Geometry check sheet. Reference: the model listing, model coordinates, mm. A direction names the side the tool comes from. Round coordinates to 2 decimals unless told otherwise and drop trailing zeros. Order: outer loops, then holes, each group sorted by start corner. A loop starts at its lowest first (then second) coordinate and runs counter-clockwise, first axis right, second up.
```python
from build123d import *

# Parameters (mm, degrees)
F1_DEPTH = 6


with BuildPart() as f1:
    # F0 (on Top) → F1 (new body)
    with BuildSketch(Plane.XY):
        with BuildLine():
            Line((38, 4), (-38, 4))
            ThreePointArc((-38, 4), (-42, 0), (-38, -4))
            Line((-38, -4), (38, -4))
            Line((38, -4), (42, 0))
            Line((42, 0), (38, 4))
        make_face()
        with BuildLine():
            ThreePointArc((-33.612533, 2.35), (-32.899958, 1.269741), (-32.65, 0))
            ThreePointArc((-32.65, 0), (-32.899958, -1.269741), (-33.612533, -2.35))
            ThreePointArc((-33.612533, -2.35), (-36, -3.35), (-38.387467, -2.35))
            ThreePointArc((-38.387467, -2.35), (-39.35, 0), (-38.387467, 2.35))
            ThreePointArc((-38.387467, 2.35), (-36, 3.35), (-33.612533, 2.35))
        make_face(mode=Mode.SUBTRACT)
        with BuildLine():
            ThreePointArc((-25.654792, 2.25), (-24.98467, 1.212554), (-24.75, 0))
            ThreePointArc((-24.75, 0), (-24.98467, -1.212554), (-25.654792, -2.25))
            ThreePointArc((-25.654792, -2.25), (-28, -3.25), (-30.345208, -2.25))
            ThreePointArc((-30.345208, -2.25), (-31.25, 0), (-30.345208, 2.25))
            ThreePointArc((-30.345208, 2.25), (-28, 3.25), (-25.654792, 2.25))
        make_face(mode=Mode.SUBTRACT)
        with BuildLine():
            ThreePointArc((-17.697827, 2.15), (-17.069612, 1.155564), (-16.85, 0))
            ThreePointArc((-16.85, 0), (-17.069612, -1.155564), (-17.697827, -2.15))
            ThreePointArc((-17.697827, -2.15), (-20, -3.15), (-22.302173, -2.15))
            ThreePointArc((-22.302173, -2.15), (-23.15, 0), (-22.302173, 2.15))
            ThreePointArc((-22.302173, 2.15), (-20, 3.15), (-17.697827, 2.15))
        make_face(mode=Mode.SUBTRACT)
        with BuildLine():
            ThreePointArc((-9.741682, 2.05), (-9.154796, 1.098779), (-8.95, 0))
            ThreePointArc((-8.95, 0), (-9.154796, -1.098779), (-9.741682, -2.05))
            ThreePointArc((-9.741682, -2.05), (-12, -3.05), (-14.258318, -2.05))
            ThreePointArc((-14.258318, -2.05), (-15.05, 0), (-14.258318, 2.05))
            ThreePointArc((-14.258318, 2.05), (-12, 3.05), (-9.741682, 2.05))
        make_face(mode=Mode.SUBTRACT)
        with BuildLine():
            ThreePointArc((-1.786406, 1.95), (-1.240235, 1.042208), (-1.05, 0))
            ThreePointArc((-1.05, 0), (-1.240235, -1.042208), (-1.786406, -1.95))
            ThreePointArc((-1.786406, -1.95), (-4, -2.95), (-6.213594, -1.95))
            ThreePointArc((-6.213594, -1.95), (-6.95, 0), (-6.213594, 1.95))
            ThreePointArc((-6.213594, 1.95), (-4, 2.95), (-1.786406, 1.95))
        make_face(mode=Mode.SUBTRACT)
        with BuildLine():
            ThreePointArc((6.167948, 1.85), (6.674056, 0.985862), (6.85, 0))
            ThreePointArc((6.85, 0), (6.674056, -0.985862), (6.167948, -1.85))
            ThreePointArc((6.167948, -1.85), (4, -2.85), (1.832052, -1.85))
            ThreePointArc((1.832052, -1.85), (1.15, 0), (1.832052, 1.85))
            ThreePointArc((1.832052, 1.85), (4, 2.85), (6.167948, 1.85))
        make_face(mode=Mode.SUBTRACT)
        with BuildLine():
            ThreePointArc((14.12132, 1.75), (14.588062, 0.92975), (14.75, 0))
            ThreePointArc((14.75, 0), (14.588062, -0.92975), (14.12132, -1.75))
            ThreePointArc((14.12132, -1.75), (12, -2.75), (9.87868, -1.75))
            ThreePointArc((9.87868, -1.75), (9.25, 0), (9.87868, 1.75))
            ThreePointArc((9.87868, 1.75), (12, 2.75), (14.12132, 1.75))
        make_face(mode=Mode.SUBTRACT)
        with BuildLine():
            ThreePointArc((22.073644, 1.65), (22.501765, 0.873883), (22.65, 0))
            ThreePointArc((22.65, 0), (22.501765, -0.873883), (22.073644, -1.65))
            ThreePointArc((22.073644, -1.65), (20, -2.65), (17.926356, -1.65))
            ThreePointArc((17.926356, -1.65), (17.35, 0), (17.926356, 1.65))
            ThreePointArc((17.926356, 1.65), (20, 2.65), (22.073644, 1.65))
        make_face(mode=Mode.SUBTRACT)
        with BuildLine():
            ThreePointArc((30, 1.5), (30.371708, 0.790569), (30.5, 0))
            ThreePointArc((30.5, 0), (30.371708, -0.790569), (30, -1.5))
            ThreePointArc((30, -1.5), (28, -2.5), (26, -1.5))
            ThreePointArc((26, -1.5), (25.5, 0), (26, 1.5))
            ThreePointArc((26, 1.5), (28, 2.5), (30, 1.5))
        make_face(mode=Mode.SUBTRACT)
        with BuildLine():
            ThreePointArc((37.922498, 1.445), (38.281188, 0.761714), (38.405, 0))
            ThreePointArc((38.405, 0), (38.281188, -0.761714), (37.922498, -1.445))
            ThreePointArc((37.922498, -1.445), (36, -2.405), (34.077502, -1.445))
            ThreePointArc((34.077502, -1.445), (33.595, 0), (34.077502, 1.445))
            ThreePointArc((34.077502, 1.445), (36, 2.405), (37.922498, 1.445))
        make_face(mode=Mode.SUBTRACT)
        with BuildLine():
            Line((-38.387467, 2.35), (-33.612533, 2.35))
            ThreePointArc((-33.612533, 2.35), (-36, 3.35), (-38.387467, 2.35))
        make_face()
        with BuildLine():
            ThreePointArc((-38.387467, -2.35), (-36, -3.35), (-33.612533, -2.35))
            Line((-33.612533, -2.35), (-38.387467, -2.35))
        make_face()
        with BuildLine():
            Line((-30.345208, 2.25), (-25.654792, 2.25))
            ThreePointArc((-25.654792, 2.25), (-28, 3.25), (-30.345208, 2.25))
        make_face()
        with BuildLine():
            ThreePointArc((-30.345208, -2.25), (-28, -3.25), (-25.654792, -2.25))
            Line((-25.654792, -2.25), (-30.345208, -2.25))
        make_face()
        with BuildLine():
            Line((-22.302173, 2.15), (-17.697827, 2.15))
            ThreePointArc((-17.697827, 2.15), (-20, 3.15), (-22.302173, 2.15))
        make_face()
        with BuildLine():
            ThreePointArc((-22.302173, -2.15), (-20, -3.15), (-17.697827, -2.15))
            Line((-17.697827, -2.15), (-22.302173, -2.15))
        make_face()
        with BuildLine():
            Line((-14.258318, 2.05), (-9.741682, 2.05))
            ThreePointArc((-9.741682, 2.05), (-12, 3.05), (-14.258318, 2.05))
        make_face()
        with BuildLine():
            ThreePointArc((-14.258318, -2.05), (-12, -3.05), (-9.741682, -2.05))
            Line((-9.741682, -2.05), (-14.258318, -2.05))
        make_face()
        with BuildLine():
            Line((-6.213594, 1.95), (-1.786406, 1.95))
            ThreePointArc((-1.786406, 1.95), (-4, 2.95), (-6.213594, 1.95))
        make_face()
        with BuildLine():
            ThreePointArc((-6.213594, -1.95), (-4, -2.95), (-1.786406, -1.95))
            Line((-1.786406, -1.95), (-6.213594, -1.95))
        make_face()
        with BuildLine():
            Line((1.832052, 1.85), (6.167948, 1.85))
            ThreePointArc((6.167948, 1.85), (4, 2.85), (1.832052, 1.85))
        make_face()
        with BuildLine():
            ThreePointArc((1.832052, -1.85), (4, -2.85), (6.167948, -1.85))
            Line((6.167948, -1.85), (1.832052, -1.85))
        make_face()
        with BuildLine():
            Line((9.87868, 1.75), (14.12132, 1.75))
            ThreePointArc((14.12132, 1.75), (12, 2.75), (9.87868, 1.75))
        make_face()
        with BuildLine():
            ThreePointArc((9.87868, -1.75), (12, -2.75), (14.12132, -1.75))
            Line((14.12132, -1.75), (9.87868, -1.75))
        make_face()
        with BuildLine():
            Line((17.926356, 1.65), (22.073644, 1.65))
            ThreePointArc((22.073644, 1.65), (20, 2.65), (17.926356, 1.65))
        make_face()
        with BuildLine():
            ThreePointArc((17.926356, -1.65), (20, -2.65), (22.073644, -1.65))
            Line((22.073644, -1.65), (17.926356, -1.65))
        make_face()
        with BuildLine():
            Line((26, 1.5), (30, 1.5))
            ThreePointArc((30, 1.5), (28, 2.5), (26, 1.5))
        make_face()
        with BuildLine():
            ThreePointArc((26, -1.5), (28, -2.5), (30, -1.5))
            Line((30, -1.5), (26, -1.5))
        make_face()
        with BuildLine():
            Line((34.077502, 1.445), (37.922498, 1.445))
            ThreePointArc((37.922498, 1.445), (36, 2.405), (34.077502, 1.445))
        make_face()
        with BuildLine():
            ThreePointArc((34.077502, -1.445), (36, -2.405), (37.922498, -1.445))
            Line((37.922498, -1.445), (34.077502, -1.445))
        make_face()
    extrude(amount=F1_DEPTH)


solid = f1.part
```
(1) Sectioned sample at B-B, the plane z = 3.15. Give the number of separate pieces and of enclosed holes in the cut face, and give its area (3 significant figures).
Returned:
separate pieces: 1
enclosed holes: 10
area: 444 mm2
(2) Material ranges on line 1 (Y direction, x = -20, z = 4.85); line 2 (Y direction, x = 22, z = 1.2); line 3 (X direction, y = 3.25, z = 1), recorded low to high.
Returned:
line 1: y = -4 to -2.15, 2.15 to 4
line 2: y = -4 to -1.65, 1.65 to 4
line 3: x = -40.33 to 38.75
(3) Sectioned sample at A-A, the plane x = -27.5. Record the cut outline in (y, z), and give its area (3 significant figures).
Returned:
outline: (-4, 0) - (-2.25, 0) - (-2.25, 6) - (-4, 6) - close; (2.25, 0) - (4, 0) - (4, 6) - (2.25, 6) - close
area: 21.0 mm2
(4) Draft check along Y on faces 3 (the flat face through (-1, -4, 3)), 4 (the flat face through (-12, 2.05, 3)), 5 (the flat face through (-0.6, 0.1, 6)). Enter one of: released by +Y, released by -Y, zero draft, split by the parting line, or undercut.
Returned:
face 3: released by -Y
face 4: undercut
face 5: zero draft
(5) Set-up check for faces 1 (the flat face through (-0.6, 0.1, 0)), 2 (the flat face through (-28, 2.25, 3)): record each of +Z, -Z, +X, -X, +Y, -Y from which the full face is reachable in a straight line by a thin tool's end or side.
Returned:
face 1: -Z, +X, -X, +Y, -Y
face 2: +Z, -Z
